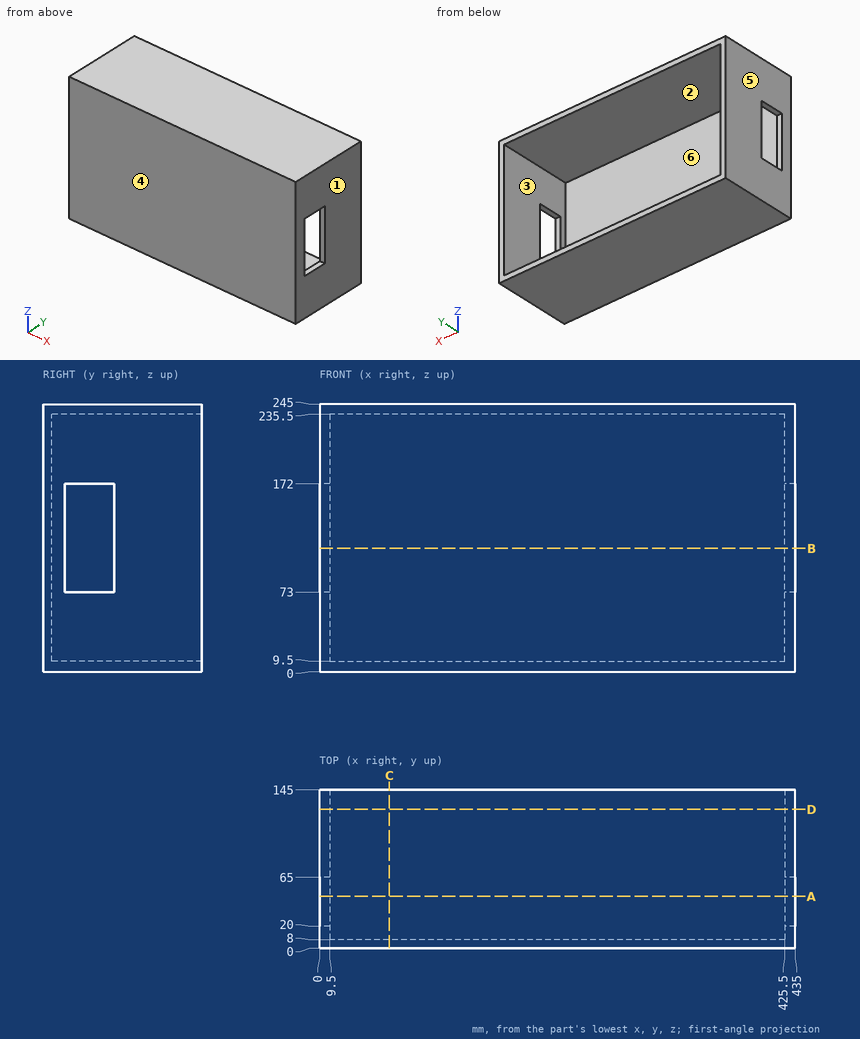
Geometry check sheet. Reference: drawing and pictorial views, mm from the part's lowest x, y, z. A direction names the side the tool comes from. Round coordinates to 2 decimals unless told otherwise and drop trailing zeros. Loops run counter-clockwise (first coordinate to the right, second up) from the corner with the lowest first, then second, coordinate; pieces in that order, holes last. Notation, with made-up numbers: (-21, 6) - (-3, 6) arc R25 ccw to (-3, 30) - close; hole circle Ø8 at (-14.75, 7). An arc over 180 degrees is marked (long way). Answer as CSV lines item,"result".
(1) Material ranges on line 1 along X through (y, z) = (89.5, 135); line 2 along Z through (x, y) = (282, 34); line 3 along Y through (x, z) = (349, 69), recorded low to high.
Output values:
line 1,"x = 0 to 9.5, 425.5 to 435"
line 2,"z = 0 to 9.5, 235.5 to 245"
line 3,"y = 0 to 8"
(2) Cross-section at D-D, the plane y = 127. Enter the section's corners in (x, z), and give its area (3 significant figures).
Output values:
outline,"(0, 0) - (435, 0) - (435, 245) - (0, 245) - close; hole (9.5, 9.5) - (425.5, 9.5) - (425.5, 235.5) - (9.5, 235.5) - close"
area,"12,600 mm²"
(3) Release check for a two-part mould opening along X. For the marked faces 3, 4, 5 and 6 record: released by +X, released by -X, zero draft, split by the parting line, or undercut.
Output values:
face 3,"undercut"
face 4,"zero draft"
face 5,"released by -X"
face 6,"undercut"
(4) Depth check by flat-ended pin: pin 1 Ø2 at (x, z) = (151.5, 45) entering from +Y. Enter the tip coordinate at first touch or a pass-through.
Output values:
pin 1,"stops at y = 8"
(5) Set-up check for the marked faces 1 and 2: record each of +Z, -Z, +X, -X, +Y, -Y from which the full face is reachable in a straight line by a thin tool's end or side.
Output values:
face 1,"+Z, -Z, +X, +Y, -Y"
face 2,"+Y"
(6) Cross-section at A-A, the plane y = 47.5. Enter the section's corners in (x, z), and give its area (3 significant figures).
Output values:
outline,"(0, 0) - (435, 0) - (435, 73) - (425.5, 73) - (425.5, 9.5) - (9.5, 9.5) - (9.5, 73) - (0, 73) - close; (0, 172) - (9.5, 172) - (9.5, 235.5) - (425.5, 235.5) - (425.5, 172) - (435, 172) - (435, 245) - (0, 245) - close"
area,"10,700 mm²"
(7) Cross-section at B-B, the plane z = 113. Enter the section's corners in (x, y).
Output values:
outline,"(0, 0) - (435, 0) - (435, 20) - (425.5, 20) - (425.5, 8) - (9.5, 8) - (9.5, 20) - (0, 20) - close; (0, 65) - (9.5, 65) - (9.5, 145) - (0, 145) - close; (425.5, 65) - (435, 65) - (435, 145) - (425.5, 145) - close"
(8) Cross-section at C-C, the plane x = 64. Enter the section's corners in (y, z).
Output values:
outline,"(0, 0) - (145, 0) - (145, 9.5) - (8, 9.5) - (8, 235.5) - (145, 235.5) - (145, 245) - (0, 245) - close"
